Autodesk Inventor part; units mm, degrees
ref_plane "YZ Plane" through (0, 0, 0) normal (1, 0, 0) x (0, 1, 0)
ref_plane "XZ Plane" through (0, 0, 0) normal (0, 1, 0) x (-1, 0, 0)
ref_plane "XY Plane" through (0, 0, 0) normal (0, 0, 1) x (1, 0, 0)
sketch "Sketch1" plane through (0, 0, 0) normal (0, 1, 0) x (-1, 0, 0)
  line L0 (600, 0) -> (600, -30)
  arc A0 (542.1993, -124.4078) -> (600, -30) centre (494, -30) ccw
  arc A1 (20, -250) -> (542.1993, -124.4078) centre (20, 898.4211) ccw
  line L1 (0, 0) -> (0, -191.6842)
  arc A2 (20, -244) -> (539.4711, -119.0639) centre (20, 898.4211) ccw
  arc A3 (539.4711, -119.0639) -> (594, -30) centre (494, -30) ccw
  line L2 (594, -30) -> (594, 0)
  line L3 (594, 0) -> (600, 0)
  line L4 (0, -244) -> (0, -250)
  line L5 (0, -250) -> (20, -250)
  line L6 (0, -244) -> (20, -244)
  point P0 (0, 0)
  point P1 (0, -163.7009)
  point P2 (0, -169.7009)
  dimension "d1" = 30
  dimension "d3" = 1148.421
  dimension "d11" = 1188
  dimension "d12" = 250
  dimension "d13" = 6
  dimension "d14" = 40
  dimension "d15" = 100
revolve "Revolution1" add sketch "Sketch1" angle 360 about axis through (0, 0, 0) along (0, 0, -1)
sketch "Sketch2" plane through (0, 0, 0) normal (0, 0, 1) x (1, 0, 0)
  circle A0 centre (0, 0) radius 16.75
  dimension "d8" = 33.5
extrude "Extrusion1" cut sketch "Sketch2" against normal through all
properties part number "PRS 1604 dished head_D1200"
Geometry: final body of the model. Coordinates: model frame, mm. A direction names the side the tool comes from. Give positions to 0.01 mm unless a question says otherwise; leave off trailing zeros. Answer as a JSON object with one key per item and string values.
1. Contact query for flat-ended pins moving along their axis: pin 1 (12 mm diameter, centred on x = 9.5, y = 10, fed in from +Z); pin 2 (12 mm diameter, centred on x = -61.5, y = -89, fed in from -Z); pin 3 (1 mm diameter, centred on x = 173, z = -116, fed in from -Y). Output: stop coordinate, or through.
Ans:
{"pin 1": "stops at z = -244", "pin 2": "stops at z = -247.06", "pin 3": "stops at y = -529.11"}
2. Access query for faces 4 (the flat face through (12, -12, -250)), 5 (the cylindrical face through (77.327, -588.945, -14.79)). Directions: +Z, -Z, +X, -X, +Y, -Y. A direction counts if a zero-diameter tool reaches every point of the face in a straight line with its end or side. Return the directions, or none.
Ans:
{"face 4": "-Z, +X, -X, +Y, -Y", "face 5": "+Z"}
3. Mould query, pull axis Y, two halves, no side actions, for faces 1 (the flat face through (12, -12, -244)), 2 (the flat face through (581, 136, 0)), 3 (the cylindrical face through (78.108, 594.894, -15.21)). Classes: pulls with the +Y half, pulls with the -Y half, needs draft (parallel to the pull), parting line crosses it, or undercut.
Ans:
{"face 1": "undercut", "face 2": "needs draft", "face 3": "parting line crosses it"}
4. Ray query, probe 1 along Y at (x, z) = (-250.5, -16.5); probe 2 along Y at (x, z) = (-25.5, -141.5); probe 3 along Z at (x, y) = (-228, -148). Return the intervals inside material, ascending. Write a range as from..to.
Ans:
{"probe 1": "y = -545.21..-538.6, 538.6..545.21", "probe 2": "y = -506.63..-492.3, 492.3..506.63", "probe 3": "z = -222.05..-215.9"}
